Read the model definition and answer for the solid it produces. Units are mm, in the model's axes. A direction names the side the tool comes from. Coordinates: 2 decimals unless noted, no trailing zeros. Write each loop counter-clockwise with the first axis right and the second up, starting at its lowest first coordinate (ties: lowest second). Pieces come first, ordered by that corner, then holes.
(1) Section B-B on y = 18 is taken. Write down the section's boundary in (x, z).
(2) Which of the six approach directions +Z, -Z, +X, -X, +Y, -Y give full straight-line access (tool end or side, diameter ignored) to faces 5 (the conical face through (-19.712, -15.136, 17.624)), 6 (the flat face through (1, -27, 0))?
(3) Find the intervals of material crossed by probe 1 along Z at (x, y) = (-19.85, -18), in increasing order.
(4) Section A-A on x = 3 is taken. Write down the section's boundary in (y, z), then the cut area to 3 significant figures.
(5) Given pin 1 (2 mm diameter, centred on x = 5, z = 16.5, fed in from +Y); pin 2 (17 mm diameter, centred on y = -9.5, z = 1, fed in from +X); pin 3 (3.5 mm diameter, centred on y = -18, z = 18, fed in from +X); pin 4 (9 mm diameter, centred on y = -18, z = -18, fed in from +X), each flat-ended and moving along its own axis, determine where each tip first touches the part or whether it passes through.
(6) Section C-C on z = 18 is taken. Write down the section's boundary in (x, y).
(7) The mould has two halves that part along X. Classify faces 1 (the flat face through (-20, 0, 0)), 2 (the flat face through (-17, 1, 0)), 3 (the cylindrical face through (0.6, -28.5, 23.2)), 4 (the flat face through (-18, -11, -30)): +X half, -X half, draft (parallel to the pull), parting line (faces both ways), or undercut.
(8) Section D-D on y = -9 is taken. Write down the section's boundary in (x, z).
from build123d import *

# Parameters (mm, degrees)
DODANIE_WYCI_GNI_CIE1_DEPTH                        = 30
DODANIE_WYCI_GNI_CIE1_DEPTH_BACK                   = 30
SZKIC1_W                                           = 40
SZKIC1_H                                           = 60
SZKIC2_W                                           = 37
SZKIC2_H                                           = 57
WYTNIJ_WYCI_GNI_CIE1_DEPTH                         = 71
SZKIC3_R                                           = 4
WYTNIJ_WYCI_GNI_CIE2_DEPTH                         = 40
POG_BIENIE_STO_KOWE_POD_M5_WKR_T_Z_BEM_D           = 5.5
POG_BIENIE_STO_KOWE_POD_M5_WKR_T_Z_BEM_DEPTH       = 10
POG_BIENIE_STO_KOWE_POD_M5_WKR_T_Z_BEM_CSINK_D     = 11.2
POG_BIENIE_STO_KOWE_POD_M5_WKR_T_Z_BEM_CSINK_ANGLE = 90
POG_BIENIE_STO_KOWE_POD_M5_WKR_T_Z_BEM_TIP         = 1.652366702
ZAOKR_GLENIE1_R                                    = 5


with BuildPart() as part:
    # Szkic1 → Dodanie-wyci_gni_cie1 (new, two sides: drawn at the far end of the back side and taken through both)
    with BuildSketch(Plane.XY.offset(-DODANIE_WYCI_GNI_CIE1_DEPTH_BACK)):
        Rectangle(SZKIC1_W, SZKIC1_H)
    extrude(amount=DODANIE_WYCI_GNI_CIE1_DEPTH + DODANIE_WYCI_GNI_CIE1_DEPTH_BACK)

    # Szkic2 → Wytnij-wyci_gni_cie1 (cut, through all)
    with BuildSketch(Plane.XY.offset(30)):
        with Locations((1.5, 1.5)):
            Rectangle(SZKIC2_W, SZKIC2_H)
    extrude(amount=-WYTNIJ_WYCI_GNI_CIE1_DEPTH, mode=Mode.SUBTRACT)

    # Szkic3 → Wytnij-wyci_gni_cie2 (cut)
    with BuildSketch(Plane(origin=(0, -30, 0), x_dir=(-1, 0, 0), z_dir=(0, -1, 0))):
        with Locations(Location((-3, -20, 0), (0, 0, 90))):
            Circle(SZKIC3_R)
        with Locations(Location((-3, 20, 0), (0, 0, 180))):
            Circle(SZKIC3_R)
    extrude(amount=-WYTNIJ_WYCI_GNI_CIE2_DEPTH, mode=Mode.SUBTRACT)

    # Pog_bienie sto_kowe pod M5 Wkr_t z _bem
    with Locations(Plane(origin=(-17, 0, 0), x_dir=(0, 0, -1), z_dir=(1, 0, 0))):
        with Locations((-18, 18), (18, 18), (18, -18), (-18, -18)):
            CounterSinkHole(POG_BIENIE_STO_KOWE_POD_M5_WKR_T_Z_BEM_D / 2, POG_BIENIE_STO_KOWE_POD_M5_WKR_T_Z_BEM_CSINK_D / 2, depth=POG_BIENIE_STO_KOWE_POD_M5_WKR_T_Z_BEM_DEPTH, counter_sink_angle=POG_BIENIE_STO_KOWE_POD_M5_WKR_T_Z_BEM_CSINK_ANGLE)
            with Locations((0, 0, -(POG_BIENIE_STO_KOWE_POD_M5_WKR_T_Z_BEM_DEPTH + POG_BIENIE_STO_KOWE_POD_M5_WKR_T_Z_BEM_TIP / 2))):  # 118° drill point
                Cone(0, POG_BIENIE_STO_KOWE_POD_M5_WKR_T_Z_BEM_D / 2, POG_BIENIE_STO_KOWE_POD_M5_WKR_T_Z_BEM_TIP, mode=Mode.SUBTRACT)

    # Zaokr_glenie1
    zaokr_glenie1_edges = [part.edges().sort_by_distance(p)[0] for p in [
        (20, -28.5, 30),
        (-18.5, 30, 30),
        (-18.5, 30, -30),
        (20, -28.5, -30),
    ]]
    fillet(zaokr_glenie1_edges, radius=ZAOKR_GLENIE1_R)


solid = part.part
Response:
1. outline: (-20, -30) - (-17, -30) - (-17, -23.6) - (-19.85, -20.75) - (-20, -20.75) - close; (-20, -15.25) - (-19.85, -15.25) - (-17, -12.4) - (-17, 12.4) - (-19.85, 15.25) - (-20, 15.25) - close; (-20, 20.75) - (-19.85, 20.75) - (-17, 23.6) - (-17, 30) - (-20, 30) - close
2. face 5: +X
2. face 6: +Z, -Z, +X, +Y
3. probe 1: z = -30 to -20.75, -15.25 to 15.25, 20.75 to 30
4. outline: (-30, -30) - (-27, -30) - (-27, -24) - (-30, -24) - close; (-30, -16) - (-27, -16) - (-27, 16) - (-30, 16) - close; (-30, 24) - (-27, 24) - (-27, 30) - (-30, 30) - close
4. area: 132 mm2
5. pin 1: stops at y = -27
5. pin 2: stops at x = -17
5. pin 3: passes through
5. pin 4: stops at x = -18.1
6. outline: (-20, -30) - (-0.46, -30) - (-0.46, -27) - (-17, -27) - (-17, -23.6) - (-19.85, -20.75) - (-20, -20.75) - close; (-20, -15.25) - (-19.85, -15.25) - (-17, -12.4) - (-17, 12.4) - (-19.85, 15.25) - (-20, 15.25) - close; (-20, 20.75) - (-19.85, 20.75) - (-17, 23.6) - (-17, 30) - (-20, 30) - close; (6.46, -30) - (20, -30) - (20, -27) - (6.46, -27) - close
7. face 1: -X half
7. face 2: +X half
7. face 3: undercut
7. face 4: draft
8. outline: (-20, -30) - (-17, -30) - (-17, 30) - (-20, 30) - close
